```python
from build123d import *

# Parameters (mm, degrees)
F1_DEPTH = 31.75
F2_R     = 1.5875
F3_DEPTH = 3.048
F4_R     = 1.27


with BuildPart() as f1:
    # F0 (on Top) → F1 (new body)
    with BuildSketch(Plane.XY):
        with BuildLine():
            ThreePointArc((8.980256, 8.980256), (0, -12.7), (-8.980256, 8.980256))
            Line((-8.980256, 8.980256), (-11.22532, 11.22532))
            ThreePointArc((-11.22532, 11.22532), (-14.666588, 6.075099), (-15.875, 0))
            Line((-15.875, 0), (-15.875, -25.4))
            Line((-15.875, -25.4), (15.875, -25.4))
            Line((15.875, -25.4), (15.875, 0))
            ThreePointArc((15.875, 0), (14.666588, 6.075099), (11.22532, 11.22532))
            Line((11.22532, 11.22532), (8.980256, 8.980256))
        make_face()
    extrude(amount=F1_DEPTH)

    # F2 (on face) → F3 (cut)
    with BuildSketch(Plane.XZ.offset(25.4)):
        with Locations((-12.7, 28.575)):
            Circle(F2_R)
        with Locations((12.7, 28.575)):
            Circle(F2_R)
        with Locations((12.7, 3.175)):
            Circle(F2_R)
        with Locations((-12.7, 3.175)):
            Circle(F2_R)
    extrude(amount=-F3_DEPTH, mode=Mode.SUBTRACT)

    # F4
    f4_edges = [f1.edges().sort_by_distance(p)[0] for p in [
        (-15.875, -12.7, 31.75),
        (0, -12.7, 31.75),
        (15.875, -12.7, 31.75),
        (10.102788, 10.102788, 0),
        (0, -12.7, 0),
        (-10.102788, 10.102788, 0),
        (-14.666588, 6.075099, 0),
        (-15.875, -12.7, 0),
        (0, -25.4, 0),
        (15.875, -12.7, 0),
        (14.666588, 6.075099, 0),
        (-8.980256, 8.980256, 15.875),
        (-11.22532, 11.22532, 15.875),
        (-10.102788, 10.102788, 31.75),
        (11.22532, 11.22532, 15.875),
        (8.980256, 8.980256, 15.875),
        (10.102788, 10.102788, 31.75),
    ]]
    fillet(f4_edges, radius=F4_R)


solid = f1.part
```
Verification items for the finished model (mm, model axes). A direction names the side the tool comes from. Coordinates: 2 decimals unless noted, no trailing zeros. Loops run counter-clockwise (first coordinate to the right, second up) from the corner with the lowest first, then second, coordinate; pieces in that order, holes last. Notation, with made-up numbers: (74.5, 84.5) - (92.5, 84.5) arc R18 ccw to (92.5, 116.5) - close; hole circle Ø1 at (-6.5, 20.25). An arc over 180 degrees is marked (long way). Return JSON: item names as keys, results as strings.
1. Tool access check on faces 1 (the cylindrical face through (-10.322, 9.81, 0.382)), 2 (the cylindrical face through (9.466, 8.984, 16.079)), 3 (the cylindrical face through (10.316, 9.804, 31.368)), 4 (the flat face through (13, -22.352, 3)). Record the directions out of +Z, -Z, +X, -X, +Y, -Y that give a thin tool (end or side, any length) a straight path to the whole face; none if there is none.
Established:
{"face 1": "-Z, +Y", "face 2": "+Z, -Z", "face 3": "+Z, +Y", "face 4": "-Y"}
2. Go/stop test with flat-tipped pins: pin 1 (5 mm diameter, centred on x = -4, z = 21, fed in from +Y); pin 2 (1 mm diameter, centred on x = 12.5, z = 28.5, fed in from -Y); pin 3 (1.9 mm diameter, centred on x = 12.7, z = 28.575, fed in from +Y). Record where each tip stops, or that it passes through.
Established:
{"pin 1": "stops at y = -10.91", "pin 2": "stops at y = -22.35", "pin 3": "stops at y = 10.53"}
3. Mould release check, pull along Z, two halves, no side actions. Record for faces 5 (the cylindrical face through (-14.89, 5.5, 15.67)), 6 (the flat face through (13, -22.352, 29)), 7 (the cylindrical face through (15.49, -12.52, 31.39)): +Z half, -Z half, draft (parallel to the pull), parting line (faces both ways), or undercut.
Established:
{"face 5": "draft", "face 6": "undercut", "face 7": "+Z half"}
4. Thickness scan on L1, parallel to Z at x = -12.7, y = -24.5; L2, parallel to X at y = -0.5, z = 14 (3 decimals); L3, parallel to Y at x = -10, z = 11. Record the ranges inside material, lowest first.
Established:
{"L1": "z = 0.06 to 1.59, 4.76 to 26.99, 30.16 to 31.75", "L2": "x = -15.875 to -12.69, 12.69 to 15.875", "L3": "y = -25.4 to -7.83, 7.83 to 10"}
5. Section check A-A, the plane x = 0. Record the boundary of the cut face in (y, z), then the cut area to 3 significant figures.
Established:
{"outline": "(-25.4, 1.27) arc R1.27 ccw to (-24.13, 0) - (-13.97, 0) arc R1.27 ccw to (-12.7, 1.27) - (-12.7, 30.48) arc R1.27 ccw to (-13.97, 31.75) - (-25.4, 31.75) - close", "area": "402 mm2"}
6. Section check B-B, the plane z = 23. Record the boundary of the cut face in (x, y) (3 decimals).
Established:
{"outline": "(-15.875, -25.4) - (15.875, -25.4) - (15.875, 0) arc R15.875 ccw to (12.159, 10.207) arc R1.27 ccw to (10.288, 10.288) - (9.837, 9.837) arc R1.27 ccw to (9.759, 8.127) arc R12.7 cw (long way) to (-9.759, 8.127) arc R1.27 ccw to (-9.837, 9.837) - (-10.288, 10.288) arc R1.27 ccw to (-12.159, 10.207) arc R15.875 ccw to (-15.875, 0) - close"}
